Part print with two shaded views. Sizes in mm from the minimum x, y, z corner. A direction names the side the tool comes from. Give positions to 0.01 mm unless a question says otherwise; leave off trailing zeros. Write each loop counter-clockwise with the first axis right and the second up, starting at its lowest first coordinate (ties: lowest second). Pieces come first, ordered by that corner, then holes. Notation, with made-up numbers: (64, 40) - (107, 40) arc R12 ccw to (107, 47) - close; hole circle Ø5 at (29.25, 81). An arc over 180 degrees is marked (long way). Answer as a JSON object with one key per item and string values.
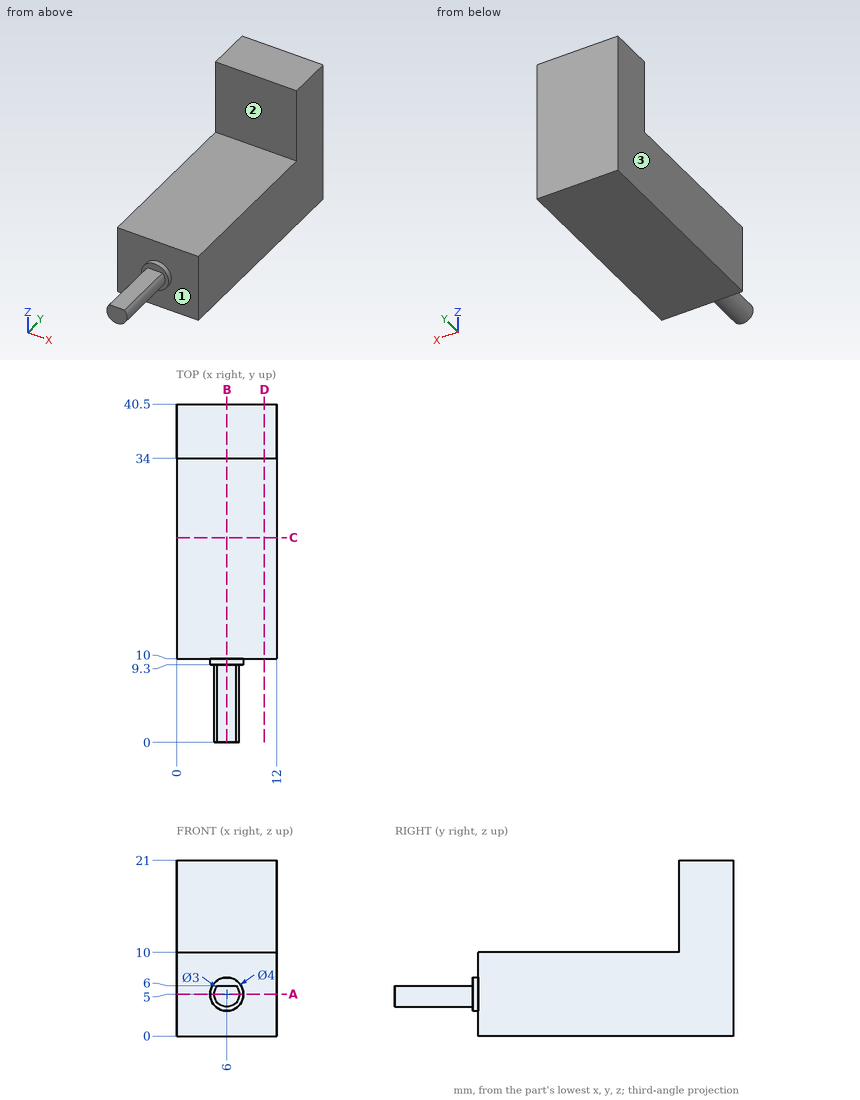
(1) Saw through at A-A, the plane z = 5. Give the cut face in (x, y), and give its area (3 significant figures).
Answer key:
{"outline": "(0, 10) - (4, 10) - (4, 9.3) - (4.5, 9.3) - (4.5, 0) - (7.5, 0) - (7.5, 9.3) - (8, 9.3) - (8, 10) - (12, 10) - (12, 40.5) - (0, 40.5) - close", "area": "397 mm²"}
(2) Probe L1, parallel to Y at x = 4, z = 5.5; L2, parallel to Z at x = 3, y = 22; L3, parallel to Y at x = 2.25, z = 13.75. List the from-to ranges inside material, lowest first. Write a range as [from, to].
Answer key:
{"L1": "y = [10, 40.5]", "L2": "z = [0, 10]", "L3": "y = [34, 40.5]"}
(3) 3-axis set-ups, long thin cutter, end or side, ignore diameter. For the marked faces 1, 2 and 3: which of +Z, -Z, +X, -X, +Y, -Y reach the whole face in a straight line?
Answer key:
{"face 1": "-Y", "face 2": "+Z, +X, -X, -Y", "face 3": "+Z, -Z, -X, +Y, -Y"}
(4) Saw through at B-B, the plane x = 6. Give the cut face in (y, z), and give its area (3 significant figures).
Answer key:
{"outline": "(0, 3.5) - (9.3, 3.5) - (9.3, 3) - (10, 3) - (10, 0) - (40.5, 0) - (40.5, 21) - (34, 21) - (34, 10) - (10, 10) - (10, 7) - (9.3, 7) - (9.3, 6) - (0, 6) - close", "area": "403 mm²"}
(5) Saw through at C-C, the plane y = 24.5. Give the cut face in (x, z), and give its area (3 significant figures).
Answer key:
{"outline": "(0, 0) - (12, 0) - (12, 10) - (0, 10) - close", "area": "120 mm²"}
(6) Flat gauge pins, fed straight in: P1, Ø4, axis at x = 10, z = 14.5, coming from the -Y side; P2, Ø3, axis at x = 4.5, y = 26.5, coming from the +Z side; P3, Ø1.8, axis at x = 6, y = 3.5, coming from the +Z side. Where does each tip first touch, or does it go through?
Answer key:
{"P1": "stops at y = 34", "P2": "stops at z = 10", "P3": "stops at z = 6"}
(7) Saw through at D-D, the plane x = 10.5. Give the cut face in (y, z).
Answer key:
{"outline": "(10, 0) - (40.5, 0) - (40.5, 21) - (34, 21) - (34, 10) - (10, 10) - close"}
